```python
from build123d import *

# Parameters (mm, degrees)
ESBO_O1_W                = 95
ESBO_O1_H                = 69
RESSALTO_EXTRUS_O1_DEPTH = 3
ESBO_O2_R                = 14
CORTE_EXTRUS_O1_DEPTH    = 59.783501087
ESBO_O4_R                = 1
CORTE_EXTRUS_O2_DEPTH    = 59.783501087
ESBO_O5_R                = 3
ESBO_O5_R_2              = 1.5
RESSALTO_EXTRUS_O2_DEPTH = 5
FILETE1_R                = 40
FILETE2_R                = 10
CORTE_EXTRUS_O3_DEPTH    = 59.919436521


with BuildPart() as part:
    # Esboço1 → Ressalto-extrusão1 (new body)
    with BuildSketch(Plane(origin=(0, 0, 0), x_dir=(1, 0, 0), z_dir=(0, 1, 0))):
        Rectangle(ESBO_O1_W, ESBO_O1_H)
    extrude(amount=RESSALTO_EXTRUS_O1_DEPTH)

    # Esboço2 → Corte-extrusão1 (cut, through all)
    with BuildSketch(Plane(origin=(0, 3, 0), x_dir=(1, 0, 0), z_dir=(0, 1, 0))):
        with Locations(Location((30.5, 0, 0), (0, 0, 270))):
            Circle(ESBO_O2_R)
    extrude(amount=-CORTE_EXTRUS_O1_DEPTH, mode=Mode.SUBTRACT)

    # Esboço4 → Corte-extrusão2 (cut, through all)
    with BuildSketch(Plane(origin=(0, 3, 0), x_dir=(1, 0, 0), z_dir=(0, 1, 0))):
        with Locations(Location((18.971497235, 25.4, 0), (0, 0, 270))):
            Circle(ESBO_O4_R)
        with Locations(Location((18.971497235, -25.4, 0), (0, 0, 90))):
            Circle(ESBO_O4_R)
        with Locations(Location((-37.5, 31.5, 0), (0, 0, 270))):
            Circle(ESBO_O4_R)
        with Locations(Location((-37.5, -31.5, 0), (0, 0, 90))):
            Circle(ESBO_O4_R)
    extrude(amount=-CORTE_EXTRUS_O2_DEPTH, mode=Mode.SUBTRACT)

    # Esboço5 → Ressalto-extrusão2 (add)
    # profile 1 of 4: a face of its own
    with BuildSketch(Plane(origin=(0, 3, 0), x_dir=(1, 0, 0), z_dir=(0, 1, 0))):
        with Locations(Location((-37.5, 31.5, 0), (0, 0, 90))):
            Circle(ESBO_O5_R)
        with Locations(Location((-37.5, 31.5, 0), (0, 0, 270))):
            Circle(ESBO_O5_R_2, mode=Mode.SUBTRACT)
    # profile 2 of 4: a face of its own
    with BuildSketch(Plane(origin=(0, 3, 0), x_dir=(1, 0, 0), z_dir=(0, 1, 0))):
        with Locations(Location((18.971497235, 25.4, 0), (0, 0, 270))):
            Circle(ESBO_O5_R)
        with Locations(Location((18.971497235, 25.4, 0), (0, 0, 270))):
            Circle(ESBO_O5_R_2, mode=Mode.SUBTRACT)
    # profile 3 of 4: a face of its own
    with BuildSketch(Plane(origin=(0, 3, 0), x_dir=(1, 0, 0), z_dir=(0, 1, 0))):
        with Locations(Location((18.971497235, -25.4, 0), (0, 0, 90))):
            Circle(ESBO_O5_R)
        with Locations(Location((18.971497235, -25.4, 0), (0, 0, 90))):
            Circle(ESBO_O5_R_2, mode=Mode.SUBTRACT)
    # profile 4 of 4: a face of its own
    with BuildSketch(Plane(origin=(0, 3, 0), x_dir=(1, 0, 0), z_dir=(0, 1, 0))):
        with Locations(Location((-37.5, -31.5, 0), (0, 0, 90))):
            Circle(ESBO_O5_R)
        with Locations(Location((-37.5, -31.5, 0), (0, 0, 90))):
            Circle(ESBO_O5_R_2, mode=Mode.SUBTRACT)
    extrude(amount=RESSALTO_EXTRUS_O2_DEPTH)

    # Filete1
    # the kernel refuses this fillet: 40 mm, written as the material it takes off along each edge
    with BuildSketch(Plane(origin=(47.5, -100, -34.5), x_dir=(0, 0, 1), z_dir=(0, 1, 0)), Plane(origin=(47.5, -100, 34.5), x_dir=(-1, 0, 0), z_dir=(0, 1, 0))) as filete1_piece_1:
        with BuildLine():
            CenterArc((FILETE1_R, -FILETE1_R), FILETE1_R, 90, 90)
            Line((0, -FILETE1_R), (0, 0))
            Line((0, 0), (FILETE1_R, 0))
        make_face()
    extrude(amount=203, mode=Mode.SUBTRACT)

    # Filete2
    filete2_edges = [part.edges().sort_by_distance(p)[0] for p in [
        (-47.5, 1.5, 34.5),
        (-47.5, 1.5, -34.5),
    ]]
    fillet(filete2_edges, radius=FILETE2_R)

    # Esboço7 → Corte-extrusão3 (cut, through all)
    with BuildSketch(Plane(origin=(0, 3, 0), x_dir=(1, 0, 0), z_dir=(0, 1, 0))):
        with BuildLine():
            Line((-31.5, 13), (8.5, 13))
            ThreePointArc((8.5, 13), (11.5, 10), (8.5, 7))
            Line((8.5, 7), (-31.5, 7))
            ThreePointArc((-31.5, 7), (-34.5, 10), (-31.5, 13))
        make_face()
        with BuildLine():
            Line((-31.5, 24.5), (8.5, 24.5))
            ThreePointArc((8.5, 24.5), (11.5, 21.5), (8.5, 18.5))
            Line((8.5, 18.5), (-31.5, 18.5))
            ThreePointArc((-31.5, 18.5), (-34.5, 21.5), (-31.5, 24.5))
        make_face()
        with BuildLine():
            Line((-31.5, -24.5), (8.5, -24.5))
            ThreePointArc((8.5, -24.5), (11.5, -21.5), (8.5, -18.5))
            Line((8.5, -18.5), (-31.5, -18.5))
            ThreePointArc((-31.5, -18.5), (-34.5, -21.5), (-31.5, -24.5))
        make_face()
        with BuildLine():
            Line((-31.5, -13), (8.5, -13))
            ThreePointArc((8.5, -13), (11.5, -10), (8.5, -7))
            Line((8.5, -7), (-31.5, -7))
            ThreePointArc((-31.5, -7), (-34.5, -10), (-31.5, -13))
        make_face()
    extrude(amount=-CORTE_EXTRUS_O3_DEPTH, mode=Mode.SUBTRACT)


solid = part.part
```
Verification items for the finished model (mm, model axes). A direction names the side the tool comes from. Give positions to 0.01 mm unless a question says otherwise; leave off trailing zeros. Order: outer loops, then holes, each group sorted by start corner. A loop starts at its lowest first (then second) coordinate and runs counter-clockwise, first axis right, second up. Notation, with made-up numbers: M 66.5,61 L 116.5,61 A17 cw 116.5,71 Z; hole C -23.75,31 d11. An arc over 180 degrees is marked long. Answer in a Markdown table with one row per item. Add a question column.
Item 1: Section check D-D, the plane z = 4. Enter the section's corners in (x, y), and give its area (3 significant figures).
Item 2: Scan lines: probe 1 along Z at (x, y) = (-13, 2.5); probe 2 along X at (y, z) = (4.6, -31.5); probe 3 along X at (y, z) = (5.65, -25.4). Record each from-to range of solid material in increasing order. Write a range as from..to.
Item 3: Section check B-B, the plane y = 6.25. Enter the section's corners in (x, z).
Item 4: Section check A-A, the plane x = -1. Enter the section's corners in (y, z), and give its area (3 significant figures).
Item 5: Gauge pin test, flat end, axial feed: pin 1 (1.5 mm diameter, centred on x = -9.5, z = 16.5, fed in from +Y). Record the tip position at first contact, or that the pin passes through.
Item 6: Section check C-C, the plane x = 36.5. Enter the section's corners in (y, z), and give its area (3 significant figures).
Item 7: Mould release check, pull along Z, two halves, no side actions. Record for faces 1 (the flat face through (-11, 2, 18.5)), 2 (the cylindrical face through (33.5, 1.5, 24.9)), 3 (the cylindrical face through (-36.51, 1.52, -31.63)), 4 (the flat face through (-47.5, 1, 0)): released by +Z, released by -Z, zero draft, split by the parting line, or undercut.
Item 8: Tool access check on faces 5 (the flat face through (18, 8, -27)), 6 (the cylindrical face through (-39.53, 5.46, -29.29)), 7 (the cylindrical face through (11.5, 1.5, 21.6)). Record the directions out of +Z, -Z, +X, -X, +Y, -Y that give a thin tool (end or side, any length) a straight path to the whole face; none if there is none.
Filled sheet:
| question | item | result |
|---|---|---|
| 1 | outline | M -47.5,0 L 17.08,0 L 17.08,3 L -47.5,3 Z; M 43.92,0 L 46.36,0 L 46.36,3 L 43.92,3 Z |
| 1 | area | 201 mm^2 |
| 2 | probe 1 | z = -34.5..-24.5, -18.5..-13, -7..7, 13..18.5, 24.5..34.5 |
| 2 | probe 2 | x = -40.5..-39, -36..-34.5 |
| 2 | probe 3 | x = 15.97..17.47, 20.47..21.97 |
| 3 | outline | C -37.5,-31.5 d6; C -37.5,31.5 d6; C 18.97,-25.4 d6; C 18.97,25.4 d6; hole C -37.5,-31.5 d3; hole C -37.5,31.5 d3; hole C 18.97,-25.4 d3; hole C 18.97,25.4 d3 |
| 4 | outline | M 0,-34.5 L 3,-34.5 L 3,-24.5 L 0,-24.5 Z; M 0,-18.5 L 3,-18.5 L 3,-13 L 0,-13 Z; M 0,-7 L 3,-7 L 3,7 L 0,7 Z; M 0,13 L 3,13 L 3,18.5 L 0,18.5 Z; M 0,24.5 L 3,24.5 L 3,34.5 L 0,34.5 Z |
| 4 | area | 135 mm^2 |
| 5 | pin 1 | stops at y = 3 |
| 6 | outline | M 0,-22.05 L 3,-22.05 L 3,-12.65 L 0,-12.65 Z; M 0,12.65 L 3,12.65 L 3,22.05 L 0,22.05 Z |
| 6 | area | 56.4 mm^2 |
| 7 | face 1 | undercut |
| 7 | face 2 | released by +Z |
| 7 | face 3 | undercut |
| 7 | face 4 | zero draft |
| 8 | face 5 | +Z, -Z, +X, -X, +Y |
| 8 | face 6 | +Y |
| 8 | face 7 | +Y, -Y |
